Build history of the part. All positions in model axes, mm. Round coordinates to 2 decimals unless told otherwise and drop trailing zeros. Order: outer loops, then holes, each group sorted by start corner. A loop starts at its lowest first (then second) coordinate and runs counter-clockwise, first axis right, second up. Notation, with made-up numbers: M 20,34 L 52,34 A20 cw 52,73 Z; hole C -20.5,50 d3. An arc over 180 degrees is marked long. Use CSV: the item, a comma, the result in double quotes.
from build123d import *

# Parameters (mm, degrees)
F0_W     = 25
F0_H     = 25
F1_DEPTH = 3
F2_D     = 2.286
F3_D     = 3.2


with BuildPart() as f1:
    # F0 (on Top) → F1 (new body)
    with BuildSketch(Plane.XY):
        Rectangle(F0_W, F0_H)
    extrude(amount=F1_DEPTH)

    # F2 (through all)
    with Locations(Plane(origin=(0, 0, 0), x_dir=(1, 0, 0), z_dir=(0, 0, -1))):
        with Locations((-6.731, 0), (6.731, 0)):
            Hole(F2_D / 2)

    # F3 (through all)
    with Locations(Plane(origin=(0, 0, 0), x_dir=(1, 0, 0), z_dir=(0, 0, -1))):
        with Locations((-9, 9), (-9, -9), (9, 9), (9, -9)):
            Hole(F3_D / 2)


solid = f1.part
(1) Drop flat-ended pins along their axis: pin 1 (4 mm diameter, centred on x = 7, y = -1, fed in from -Z); pin 2 (1.9 mm diameter, centred on x = 9, y = -9, fed in from +Z). Give the stop position or say it passes through.
Answer block:
pin 1,"stops at z = 0"
pin 2,"passes through"
(2) Two-plate mould, pull along X, no slides. Class faces 1 (the face through (-12.5, 0, 1)), 2 (the face through (0, 12.5, 1)), 3 (the face through (-8.65, -7.44, 1.52)): released by +X, released by -X, zero draft, split by the parting line, or undercut.
Answer block:
face 1,"released by -X"
face 2,"zero draft"
face 3,"undercut"
(3) Wall check: line 1 (Y direction, x = 9, z = 2.2); line 2 (Y direction, x = 8.25, z = 2.05). Give the ranges that are in metal, low to high. Write a range as from..to.
Answer block:
line 1,"y = -12.5..-10.6, -7.4..7.4, 10.6..12.5"
line 2,"y = -12.5..-10.41, -7.59..7.59, 10.41..12.5"
(4) Cut at A-A, the plane y = 0. Give the cut face in (x, z).
Answer block:
outline,"M -12.5,0 L -7.87,0 L -7.87,3 L -12.5,3 Z; M -5.59,0 L 5.59,0 L 5.59,3 L -5.59,3 Z; M 7.87,0 L 12.5,0 L 12.5,3 L 7.87,3 Z"
(5) Cut at C-C, the plane x = -9. Give the cut face in (y, z).
Answer block:
outline,"M -12.5,0 L -10.6,0 L -10.6,3 L -12.5,3 Z; M -7.4,0 L 7.4,0 L 7.4,3 L -7.4,3 Z; M 10.6,0 L 12.5,0 L 12.5,3 L 10.6,3 Z"
(6) Cut at B-B, the plane z = 1.3. Give the cut face in (x, y).
Answer block:
outline,"M -12.5,-12.5 L 12.5,-12.5 L 12.5,12.5 L -12.5,12.5 Z; hole C -9,-9 d3.2; hole C -9,9 d3.2; hole C -6.73,0 d2.29; hole C 6.73,0 d2.29; hole C 9,-9 d3.2; hole C 9,9 d3.2"
